The drawing under review shows one solid part. Ordinate dimensions are in mm from its lowest x, y, z. A direction names the side the tool comes from. Round coordinates to 2 decimals unless told otherwise and drop trailing zeros. Order: outer loops, then holes, each group sorted by start corner. A loop starts at its lowest first (then second) coordinate and runs counter-clockwise, first axis right, second up. Notation, with made-up numbers: M -18,87.25 L 37,87.25 A19 ccw 37,104.25 Z; hole C 41.5,-2 d2. An arc over 180 degrees is marked long. Answer as a JSON object with one key per item and string values.
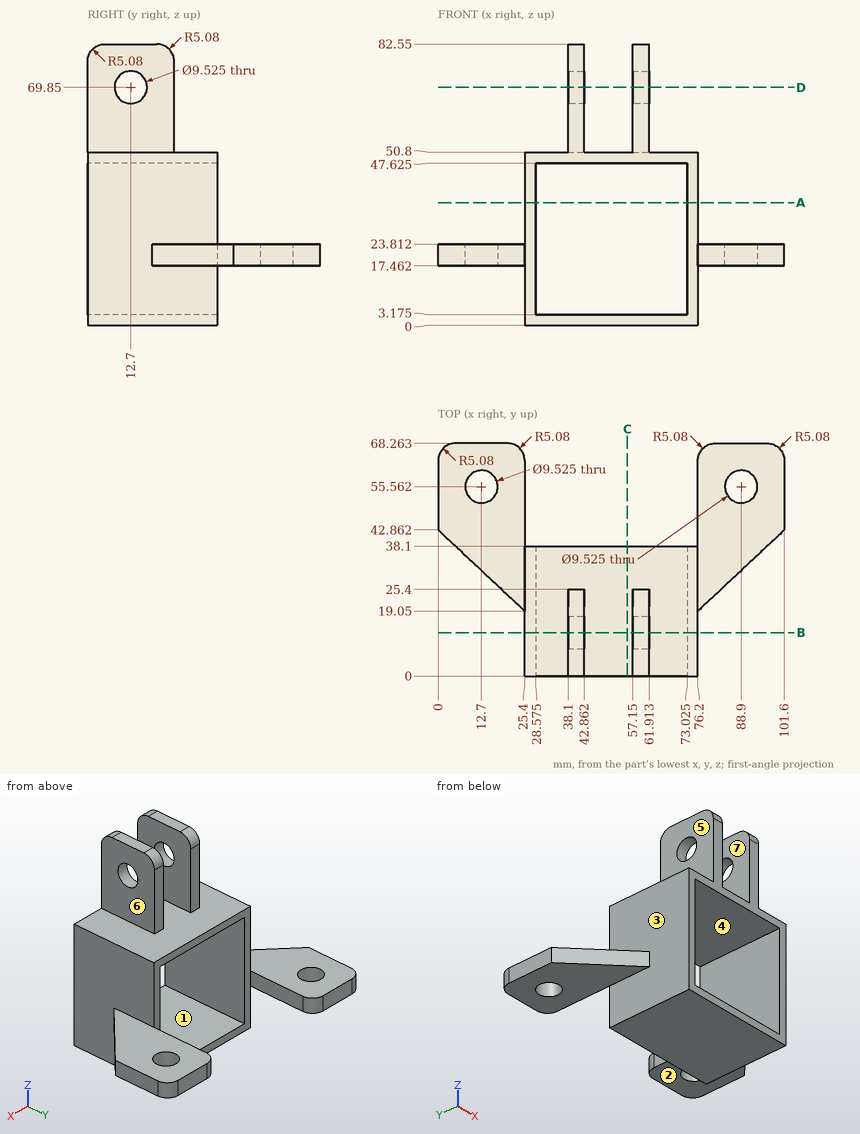
1) Add section A-A on z = 36. State the section outline as (x, y) points (1 decimal), and give its area (3 significant figures).
Geometry check:
{"outline": "M 25.4,0 L 28.6,0 L 28.6,38.1 L 25.4,38.1 Z; M 73,0 L 76.2,0 L 76.2,38.1 L 73,38.1 Z", "area": "242 mm²"}
2) Machinability: for the marked faces 4, 5, 6 and 7, which of the approach directions +Z, -Z, +X, -X, +Y, -Y give a long, thin tool a straight path to every point of the face, cutting with its end or side? Answer none if there is none.
Geometry check:
{"face 4": "+Y, -Y", "face 5": "+Z, -X, +Y, -Y", "face 6": "+Z, +X, +Y, -Y", "face 7": "+Z, +Y, -Y"}
3) Add section B-B on y = 12.7. State how many separate pieces and enclosed holes the cut face has.
Geometry check:
{"separate pieces": "3", "enclosed holes": "1"}
4) Insertion check: P1, Ø8, axis at x = 59.5, z = 44, coming from the -Y side; P2, Ø11, axis at y = 12.7, z = 69.85, coming from the +X side; P3, Ø1.4, axis at x = 41.5, z = 65.5, coming from the +Y side; P4, Ø12.5, axis at x = 92.5, y = 42, coming from the +Z side. Each pin has a flat end and moves straight along its axis. Give the tip position at first contact, or say it passes through.
Geometry check:
{"P1": "stops at y = 0", "P2": "stops at x = 61.91", "P3": "stops at y = 25.4", "P4": "stops at z = 23.81"}
5) Mouldability with a two-part tool opening along X and no side actions: class the marked faces 1, 2 and 3 as +X half, -X half, draft (parallel to the pull), parting line (faces both ways), or undercut.
Geometry check:
{"face 1": "undercut", "face 2": "draft", "face 3": "-X half"}
6) Add section D-D on z = 69.85. State the section outline as (x, y) points, and give its area (3 significant figures).
Geometry check:
{"outline": "M 38.1,0 L 42.86,0 L 42.86,7.94 L 38.1,7.94 Z; M 38.1,17.46 L 42.86,17.46 L 42.86,25.4 L 38.1,25.4 Z; M 57.15,0 L 61.91,0 L 61.91,7.94 L 57.15,7.94 Z; M 57.15,17.46 L 61.91,17.46 L 61.91,25.4 L 57.15,25.4 Z", "area": "151 mm²"}
7) Add section C-C on x = 55.5. State the section outline as (y, z) points (1 decimal), and give its area (3 significant figures).
Geometry check:
{"outline": "M 0,0 L 38.1,0 L 38.1,3.2 L 0,3.2 Z; M 0,47.6 L 38.1,47.6 L 38.1,50.8 L 0,50.8 Z", "area": "242 mm²"}
8) For L1, parallel to X at y = 16, z = 5.5 (1 decimal); L2, parallel to Y at x = 58.3, z = 69.85; L3, parallel to X at y = 13, z = 51.5, list the stretches that pass through material, from the lowest coordinate up.
Geometry check:
{"L1": "x = 25.4 to 28.6, 73 to 76.2", "L2": "y = 0 to 7.94, 17.46 to 25.4", "L3": "x = 38.1 to 42.86, 57.15 to 61.91"}
